from build123d import *

# Parameters (mm, degrees)
SKETCH_1_W                 = 160
SKETCH_1_H                 = 120
EXTRUDE_160X120_DEPTH      = 6
CUT_EXTRUDE_392_DEPTH      = 101.179838291
CUT_EXTRUDE_392_DEPTH_BACK = 101.179838291
SKETCH_2_R                 = 2.25
SKETCH_2_R_2               = 5
SKETCH_2_W                 = 20
SKETCH_2_H                 = 3.5


with BuildPart() as part:
    # 草图1 → 主板通用托盘160x120 (new body)
    with BuildSketch(Plane.XY):
        Rectangle(SKETCH_1_W, SKETCH_1_H)
    extrude(amount=EXTRUDE_160X120_DEPTH)

    # 草图2 → Cut-Extrude 392 (cut, two sides: drawn at the far end of the back side and taken through both)
    with BuildSketch(Plane.XY.offset(-CUT_EXTRUDE_392_DEPTH_BACK)):
        with Locations((-55, 0)):
            Circle(SKETCH_2_R)
        with Locations((55, 0)):
            Circle(SKETCH_2_R)
        with Locations((-35, -30)):
            Circle(SKETCH_2_R_2)
        with Locations((-35, 0)):
            Circle(SKETCH_2_R_2)
        with Locations((-35, 30)):
            Circle(SKETCH_2_R_2)
        with Locations((0, -30)):
            Circle(SKETCH_2_R_2)
        Circle(SKETCH_2_R_2)
        with Locations((0, 30)):
            Circle(SKETCH_2_R_2)
        with Locations((35, -30)):
            Circle(SKETCH_2_R_2)
        with Locations((35, 0)):
            Circle(SKETCH_2_R_2)
        with Locations((35, 30)):
            Circle(SKETCH_2_R_2)
        with Locations((-60, -48)):
            Rectangle(SKETCH_2_W, SKETCH_2_H)
        with Locations((-60, 48)):
            Rectangle(SKETCH_2_W, SKETCH_2_H)
        with Locations((60, -48)):
            Rectangle(SKETCH_2_W, SKETCH_2_H)
        with Locations((60, 48)):
            Rectangle(SKETCH_2_W, SKETCH_2_H)
    extrude(amount=CUT_EXTRUDE_392_DEPTH + CUT_EXTRUDE_392_DEPTH_BACK, mode=Mode.SUBTRACT)


solid = part.part
Verification items for the finished model (mm, model axes). A direction names the side the tool comes from. Round coordinates to 2 decimals unless told otherwise and drop trailing zeros. Loops run counter-clockwise (first coordinate to the right, second up) from the corner with the lowest first, then second, coordinate; pieces in that order, holes last. Notation, with made-up numbers: M -23,-22 L -19,-22 A33 ccw -19,8 Z; hole C 39,88.25 d1. An arc over 180 degrees is marked long. Write each question's results on one line, items separated by ' | '.
1) Scan lines: L1, parallel to Y at x = 67.5, z = 1.9; L2, parallel to Y at x = 35, z = 2.5; L3, parallel to X at y = 0, z = 3.5. Record each from-to range of solid material in increasing order. Write a range as from..to.
Checks:
L1: y = -60..-49.75, -46.25..46.25, 49.75..60 | L2: y = -60..-35, -25..-5, 5..25, 35..60 | L3: x = -80..-57.25, -52.75..-40, -30..-5, 5..30, 40..52.75, 57.25..80
2) Section check D-D on y = -30. Record the boundary of the cut face in (x, z), then the cut area to 3 significant figures.
Checks:
outline: M -80,0 L -40,0 L -40,6 L -80,6 Z; M -30,0 L -5,0 L -5,6 L -30,6 Z; M 5,0 L 30,0 L 30,6 L 5,6 Z; M 40,0 L 80,0 L 80,6 L 40,6 Z | area: 780 mm2
3) Section check A-A on x = -55. Record the boundary of the cut face in (y, z), then the cut area to 3 significant figures.
Checks:
outline: M -60,0 L -49.75,0 L -49.75,6 L -60,6 Z; M -46.25,0 L -2.25,0 L -2.25,6 L -46.25,6 Z; M 2.25,0 L 46.25,0 L 46.25,6 L 2.25,6 Z; M 49.75,0 L 60,0 L 60,6 L 49.75,6 Z | area: 651 mm2
4) Gauge pin test, flat end, axial feed: P1, Ø8, axis at x = -35, y = -30, coming from the -Z side. Record the tip position at first contact, or that the pin passes through.
Checks:
P1: passes through
5) Section check B-B on y = 0. Record the boundary of the cut face in (x, z).
Checks:
outline: M -80,0 L -57.25,0 L -57.25,6 L -80,6 Z; M -52.75,0 L -40,0 L -40,6 L -52.75,6 Z; M -30,0 L -5,0 L -5,6 L -30,6 Z; M 5,0 L 30,0 L 30,6 L 5,6 Z; M 40,0 L 52.75,0 L 52.75,6 L 40,6 Z; M 57.25,0 L 80,0 L 80,6 L 57.25,6 Z
6) Section check C-C on z = 4.3. State how many separate pieces and enclosed holes the cut face has, then the cut area to 3 significant figures.
Checks:
separate pieces: 1 | enclosed holes: 15 | area: 18,200 mm2
7) Access from +Z, -Z, +X, -X, +Y, -Y to the whole of each face (thin tool, end or side, straight path). Record for faces 4 (the flat face through (-80, -1, 3)), 5 (the flat face through (-50, 48, 3)).
Checks:
face 4: +Z, -Z, -X, +Y, -Y | face 5: +Z, -Z
8) Mould release check, pull along Y, two halves, no side actions. Record for faces 1 (the flat face through (-1, 14, 6)), 2 (the flat face through (-1, -60, 3)), 3 (the cylindrical face through (-1.08, -4.88, 2.96)): released by +Y, released by -Y, zero draft, split by the parting line, or undercut.
Checks:
face 1: zero draft | face 2: released by -Y | face 3: undercut
